Input: dimensioned drawing with shaded views. Units: mm. Origin: part minimum x, y, z. A direction names the side the tool comes from. Coordinates: 2 decimals unless noted, no trailing zeros. Order: outer loops, then holes, each group sorted by start corner. A loop starts at its lowest first (then second) coordinate and runs counter-clockwise, first axis right, second up. Notation, with made-up numbers: (81.25, 57) -> (101.25, 57) arc R21 cw to (101.25, 67) -> close; hole circle Ø3 at (70, -27.75). An arc over 180 degrees is marked (long way). Write item = value, one per line. Start each with the question number.
Item 1: Section query C-C (z = 36.3). Output: boundary loops of the cut face in (x, y), then the cut area to 3 significant figures.
Item 2: Section query A-A (x = 8). Output: boundary loops of the cut face in (y, z).
Item 3: Section query B-B (y = 37). Output: boundary loops of the cut face in (x, z) (1 decimal).
Item 4: Set-up query: the marked faces 1 and 2. Return all of +Z, -Z, +X, -X, +Y, -Y with unobstructed straight access to the full face (end or side cutting, diameter ignored); none if empty.
Item 5: Section query D-D (z = 12.5). Output: boundary loops of the cut face in (x, y) (1 decimal), then the cut area to 3 significant figures.
Item 6: Ray query, line 1 along X through (y, z) = (1, 35); line 2 along X through (y, z) = (9, 19.5). Return the intervals inside material, ascending. Write a range as [from, to].
Item 7: Contact query for flat-ended pins moving along their axis: pin 1 (19 mm diameter, centred on x = 12.5, z = 15.5, fed in from +Y); pin 2 (2.5 mm diameter, centred on y = 12.97, z = 28.58, fed in from -X) (3 decimals); pin 3 (8 mm diameter, centred on y = 25, z = 4.5, fed in from +X); pin 4 (1.4 mm diameter, centred on x = 0.5, y = 29.5, fed in from -Z). Output: stop coordinate, or through.
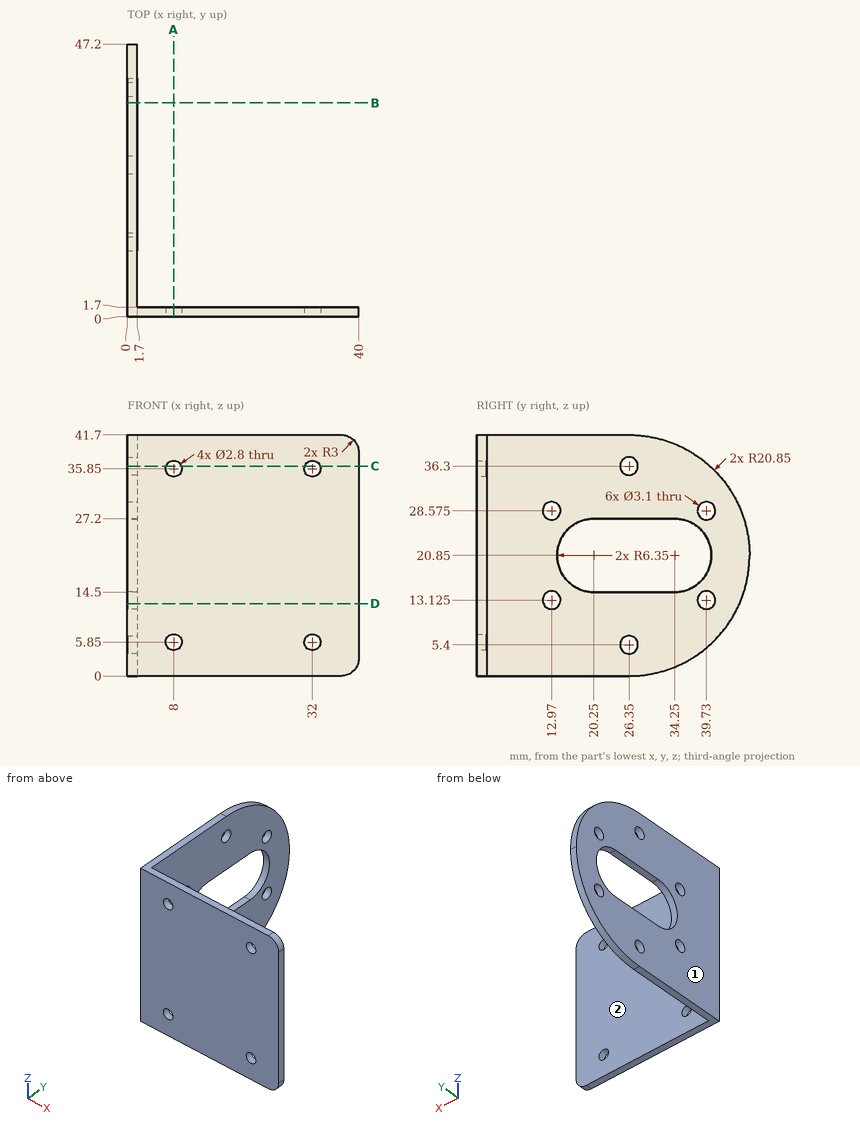
Computed:
q1.outline = (0, 0) -> (6.67, 0) -> (6.67, 1.7) -> (1.7, 1.7) -> (1.7, 24.8) -> (0, 24.8) -> close; (0, 27.9) -> (1.7, 27.9) -> (1.7, 40.35) -> (0, 40.35) -> close; (9.33, 0) -> (30.67, 0) -> (30.67, 1.7) -> (9.33, 1.7) -> close; (33.33, 0) -> (40, 0) -> (40, 1.7) -> (33.33, 1.7) -> close
q1.area = 119 mm^2
q2.outline = (0, 0) -> (1.7, 0) -> (1.7, 4.45) -> (0, 4.45) -> close; (0, 7.25) -> (1.7, 7.25) -> (1.7, 34.45) -> (0, 34.45) -> close; (0, 37.25) -> (1.7, 37.25) -> (1.7, 41.7) -> (0, 41.7) -> close
q3.outline = (0, 2.9) -> (1.7, 2.9) -> (1.7, 15.1) -> (0, 15.1) -> close; (0, 26.6) -> (1.7, 26.6) -> (1.7, 38.8) -> (0, 38.8) -> close
q4.face_1 = +Z, -Z, -X, +Y, -Y
q4.face_2 = +Z, -Z, +X, +Y
q5.outline = (0, 0) -> (40, 0) -> (40, 1.7) -> (1.7, 1.7) -> (1.7, 11.6) -> (0, 11.6) -> close; (0, 14.4) -> (1.7, 14.4) -> (1.7, 38.3) -> (0, 38.3) -> close; (0, 41.1) -> (1.7, 41.1) -> (1.7, 45.5) -> (0, 45.5) -> close
q5.area = 133 mm^2
q6.line_1 = [0, 6.89], [9.11, 30.89], [33.11, 40]
q6.line_2 = [0, 1.7]
q7.pin_1 = 1.7
q7.pin_2 = through
q7.pin_3 = 1.7
q7.pin_4 = 0.14
